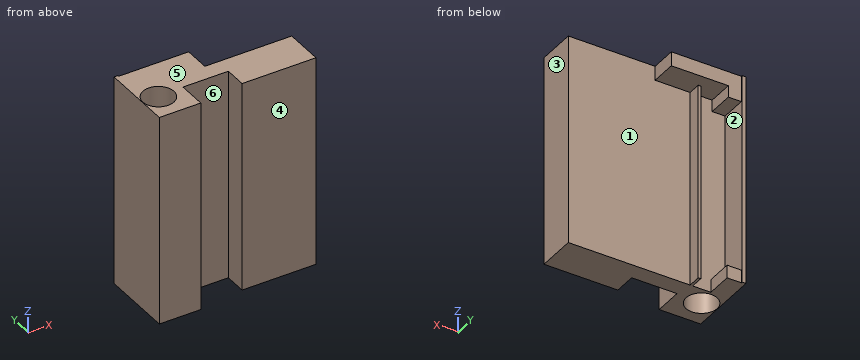
```python
from build123d import *

# Parameters (mm, degrees)
PAD_DEPTH    = 81.5
SKETCH001_R  = 6
POCKET_DEPTH = 81.501
SKETCH002_W  = 5.5
SKETCH002_H  = 5
PAD001_DEPTH = 10
SKETCH003_W  = 1
SKETCH003_H  = 81.5
PAD002_DEPTH = 5


with BuildPart() as part:
    # Sketch → Pad (new body)
    with BuildSketch(Plane.XY):
        Polygon((62, -10.5), (62, -25.5), (33.5, -25.5), (33.5, -17), (16, -17), (16, -28), (0, -28), (0, 0), (1.5, 0), (1.5, -10.5), align=None)
    extrude(amount=PAD_DEPTH)

    # Sketch001 (on Face12 of Pad) → Pocket (cut, through all)
    with BuildSketch(Plane.XY.offset(81.5)):
        with Locations((6.2, -17.5)):
            Circle(SKETCH001_R)
    extrude(amount=-POCKET_DEPTH, mode=Mode.SUBTRACT)

    # Sketch002 (on Face12 of Pocket) → Pad001 (join)
    with BuildSketch(Plane(origin=(0, -10.5, 0), x_dir=(-1, 0, 0), z_dir=(0, 1, 0))):
        with Locations((-4.25, 2.5)):
            Rectangle(SKETCH002_W, SKETCH002_H)
        Polygon((-28.5, 81.5), (-1.5, 81.5), (-1.5, 71.5), (-6.5, 71.5), (-6.5, 76), (-28.5, 76), align=None)
    extrude(amount=PAD001_DEPTH)

    # Sketch003 (on Face13 of Pad001) → Pad002 (join)
    with BuildSketch(Plane(origin=(0, -10.5, 0), x_dir=(-1, 0, 0), z_dir=(0, 1, 0))):
        with Locations((-14.5, 40.75)):
            Rectangle(SKETCH003_W, SKETCH003_H)
    extrude(amount=PAD002_DEPTH)


solid = part.part
```
Check sheet for the modelled part. Datum: model origin and axes. Units: mm. Face numbers are marked on the shaded views. A direction names the side the tool comes from. Give positions to 0.01 mm unless a question says otherwise; leave off trailing zeros. Order: outer loops, then holes, each group sorted by start corner. A loop starts at its lowest first (then second) coordinate and runs counter-clockwise, first axis right, second up. Notation, with made-up numbers: (18, 65.25) -> (50, 65.25) arc R33 cw to (50, 97.25) -> close; hole circle Ø8 at (68, 81.25). An arc over 180 degrees is marked (long way). Use CSV: the item, a comma, the result in double quotes. Start each with the question number.
1) Mould release check, pull along X, two halves, no side actions. Record for the marked faces 1, 2 and 3: released by +X, released by -X, zero draft, split by the parting line, or undercut.
2) Go/stop test with flat-tipped pins: P1, Ø4.5, axis at y = -4, z = 78.5, coming from the +X side; P2, Ø4, axis at y = -4, z = 3, coming from the +X side; P3, Ø8, axis at x = 8, y = -18.5, coming from the -Z side; P4, Ø14, axis at x = 50.5, z = 52.5, coming from the -Y side. Record where each tip stops, or that it passes through.
3) Sectioned sample at B-B, the plane x = 8. Record the boundary of the cut face in (y, z).
4) Material ranges on line 1 (Y direction, x = 6, z = 49); line 2 (Z direction, x = 5, y = -10); line 3 (X direction, y = -18.75, z = 57), recorded low to high. Write a range as from..to.
5) Sectioned sample at C-C, the plane z = 46. Record the boundary of the cut face in (x, y), plus the area to 3 significant figures.
6) Set-up check for the marked faces 4, 5 and 6: record each of +Z, -Z, +X, -X, +Y, -Y from which the full face is reachable in a straight line by a thin tool's end or side.
7) Sectioned sample at D-D, the plane y = -13.5. Record the boundary of the cut face in (x, z).
8) Sectioned sample at A-A, the plane y = -2.25. Record the boundary of the cut face in (x, z).
Recorded:
1,face 1,"zero draft"
1,face 2,"undercut"
1,face 3,"released by +X"
2,P1,"x = 28.5"
2,P2,"x = 15"
2,P3,"z = 0"
2,P4,"y = -25.5"
3,outline,"(-28, 0) -> (-23.22, 0) -> (-23.22, 81.5) -> (-28, 81.5) -> close; (-11.78, 0) -> (-10.5, 0) -> (-10.5, 76) -> (-0.5, 76) -> (-0.5, 81.5) -> (-11.78, 81.5) -> close"
4,line 1,"-28..-23.5, -11.5..-10.5"
4,line 2,"0..5, 71.5..81.5"
4,line 3,"0..0.33, 12.07..16, 33.5..62"
5,outline,"(0, -28) -> (16, -28) -> (16, -17) -> (33.5, -17) -> (33.5, -25.5) -> (62, -25.5) -> (62, -10.5) -> (15, -10.5) -> (15, -5.5) -> (14, -5.5) -> (14, -10.5) -> (1.5, -10.5) -> (1.5, 0) -> (0, 0) -> close; hole circle Ø12 at (6.2, -17.5)"
5,area,"729 mm2"
6,face 4,"+Z, -Z, +X, -Y"
6,face 5,"+Z, +X, -X, +Y, -Y"
6,face 6,"+Z, -Z, -Y"
7,outline,"(0, 0) -> (1.73, 0) -> (1.73, 81.5) -> (0, 81.5) -> close; (10.67, 0) -> (62, 0) -> (62, 81.5) -> (10.67, 81.5) -> close"
8,outline,"(0, 0) -> (7, 0) -> (7, 5) -> (1.5, 5) -> (1.5, 71.5) -> (6.5, 71.5) -> (6.5, 76) -> (28.5, 76) -> (28.5, 81.5) -> (0, 81.5) -> close"
